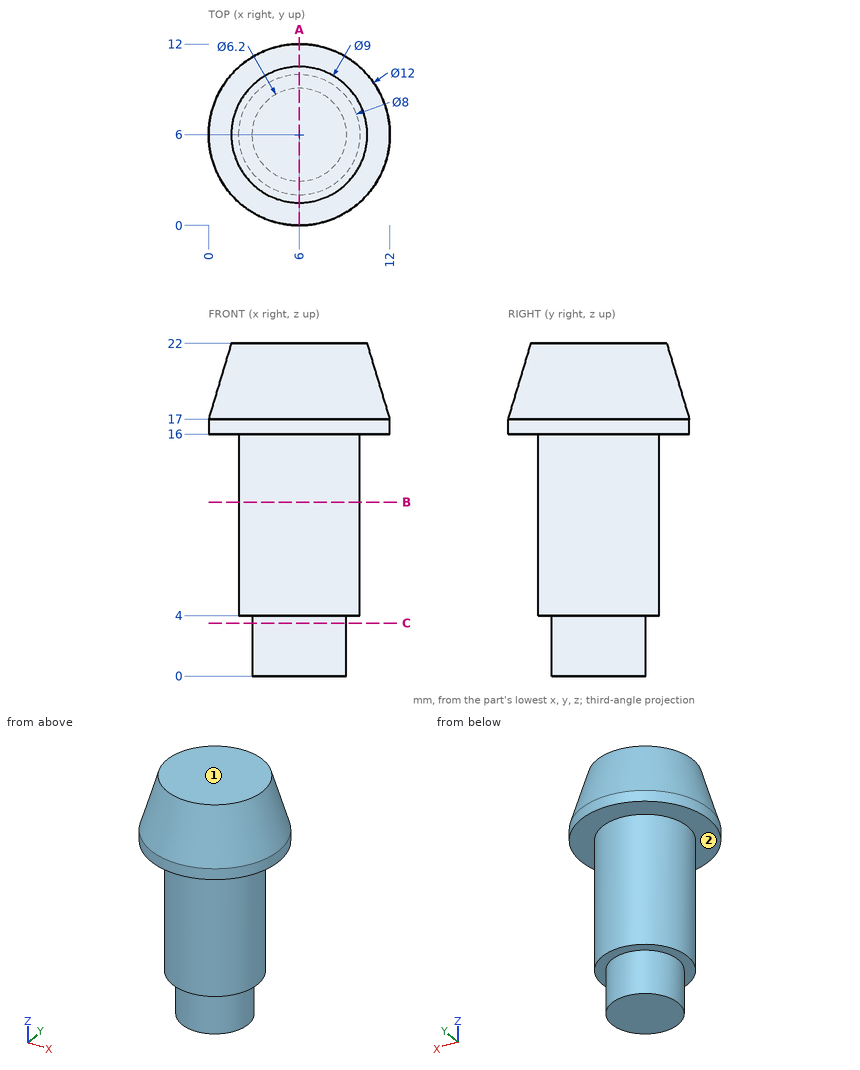
Source: three-view drawing plus pictorial views. Frame: mm from the lowest corner of the part. A direction names the side the tool comes from. Give positions to 0.01 mm unless a question says otherwise; leave off trailing zeros. Order: outer loops, then holes, each group sorted by start corner. A loop starts at its lowest first (then second) coordinate and runs counter-clockwise, first axis right, second up. Notation, with made-up numbers: M -4,11 L 19,11 A38 ccw 19,50 Z; hole C 32,76 d1. An arc over 180 degrees is marked long. One line per question, with ' | ' between items.
1) Access query for the marked faces 1 and 2. Directions: +Z, -Z, +X, -X, +Y, -Y. A direction counts if a zero-diameter tool reaches every point of the face in a straight line with its end or side. Return the directions, or none.
Filled in:
face 1: +Z, +X, -X, +Y, -Y | face 2: -Z
2) Section C-C on z = 3.5. Output: boundary loops of the cut face in (x, y).
Filled in:
outline: C 6,6 d6.2
3) Ray query, L1, parallel to Z at x = 4.25, y = 9; L2, parallel to Y at x = 11, z = 19; L3, parallel to X at y = 9.5, z = 10.75. Return the intervals inside material, ascending.
Filled in:
L1: z = 4 to 22 | L2: y = 3.96 to 8.04 | L3: x = 4.06 to 7.94
4) Section B-B on z = 11.5. Output: boundary loops of the cut face in (x, y).
Filled in:
outline: C 6,6 d8
5) Contact query for flat-ended pins moving along their axis: P1, Ø5, axis at y = 2.5, z = 9.5, coming from the -X side; P2, Ø5, axis at y = 8.5, z = 9.5, coming from the +X side. Output: stop coordinate, or through.
Filled in:
P1: stops at x = 2.13 | P2: stops at x = 10
6) Section A-A on x = 6. Output: boundary loops of the cut face in (y, z).
Filled in:
outline: M 0,16 L 2,16 L 2,4 L 2.9,4 L 2.9,0 L 9.1,0 L 9.1,4 L 10,4 L 10,16 L 12,16 L 12,17 L 10.5,22 L 1.5,22 L 0,17 Z
